Work out the finished part from the listing and answer in its coordinate system (mm). Face numbers are marked on the shaded views. Round coordinates to 2 decimals unless told otherwise and drop trailing zeros. Order: outer loops, then holes, each group sorted by start corner. A loop starts at its lowest first (then second) coordinate and runs counter-clockwise, first axis right, second up. Notation, with made-up numbers: (13, -25) -> (20, -25) arc R6 ccw to (20, -18) -> close; hole circle Ø4 at (81, -8.5). An arc over 180 degrees is marked (long way). Use one line per item in the form item = value.
```python
from build123d import *

# Parameters (mm, degrees)
REVOLVE2_ANGLE           = 7.5
SKETCH4_W                = 33.25
SKETCH4_H                = 13
CUT_EXTRUDE5_DEPTH       = 19
SKETCH7_W                = 33.25
SKETCH7_H                = 13
CUT_EXTRUDE7_DEPTH       = 19
CUT_EXTRUDE8_DEPTH       = 1799.499288206
CUT_EXTRUDE8_DEPTH_BACK  = 1799.499288206
SKETCH9_W                = 188.635889627
SKETCH9_H                = 632.041441351
CUT_EXTRUDE9_DEPTH       = 1799.499288206
CUT_EXTRUDE9_DEPTH_BACK  = 1799.499288206
SKETCH10_W               = 436.927860133
SKETCH10_H               = 1601.4752783
CUT_EXTRUDE10_DEPTH      = 143.403889156
CUT_EXTRUDE10_DEPTH_BACK = 143.403889156


with BuildPart() as part:
    # Sketch2 → Revolve2 (revolve)
    with BuildSketch(Plane.XY):
        with BuildLine():
            Line((0, 993.075249624), (0, 990.6))
            ThreePointArc((0, 990.6), (990.6, 0), (0, -990.6))
            Line((0, -990.6), (0, -993.075249624))
            ThreePointArc((0, -993.075249624), (357.30221933, -926.570869107), (666.748724276, -735.965073963))
            Line((666.748724276, -735.965073963), (742.973100692, -735.965073963))
            Line((742.973100692, -735.965073963), (742.973100692, -658.930514596))
            ThreePointArc((742.973100692, -658.930514596), (993.075236283, 0.162783709), (742.757038562, 659.174053709))
            Line((742.757038562, 659.174053709), (742.757038562, 722.715073963))
            Line((742.757038562, 722.715073963), (681.088374063, 722.715073963))
            ThreePointArc((681.088374063, 722.715073963), (366.393230651, 923.013787519), (0, 993.075249624))
        make_face()
    revolve(axis=Axis((0, 993.075249624, 0), (0, -1, 0)), revolution_arc=REVOLVE2_ANGLE)

    # Sketch4 → Cut-Extrude5 (cut)
    with BuildSketch(Plane.XZ.offset(735.965073963)):
        with Locations((705.258501449, 49.061390401)):
            Rectangle(SKETCH4_W, SKETCH4_H)
    extrude(amount=-CUT_EXTRUDE5_DEPTH, mode=Mode.SUBTRACT)

    # Sketch7 → Cut-Extrude7 (cut)
    with BuildSketch(Plane(origin=(0, 722.715073963, 0), x_dir=(-1, 0, 0), z_dir=(0, 1, 0))):
        with Locations((-714.999743141, 46.422731407)):
            Rectangle(SKETCH7_W, SKETCH7_H)
    extrude(amount=-CUT_EXTRUDE7_DEPTH, mode=Mode.SUBTRACT)

    # Sketch9 → Cut-Extrude8 (cut, two sides: drawn at the far end of the back side and taken through both)
    with BuildSketch(Plane(origin=(770.075395243, 627.042532096, 0), x_dir=(0, 0, -1), z_dir=(0.775445159402277, 0.6314149228198344, 0)).offset(-CUT_EXTRUDE8_DEPTH_BACK)):
        with Locations((-24.021749008, 516.225121034)):
            Rectangle(SKETCH9_W, SKETCH9_H)
    extrude(amount=CUT_EXTRUDE8_DEPTH + CUT_EXTRUDE8_DEPTH_BACK, mode=Mode.SUBTRACT)

    # Sketch10 → Cut-Extrude9 (cut, two sides: drawn at the far end of the back side and taken through both)
    with BuildSketch(Plane(origin=(770.075395243, 627.042532096, 0), x_dir=(0, 0, -1), z_dir=(0.775445159402277, 0.6314149228198344, 0)).offset(-CUT_EXTRUDE9_DEPTH_BACK)):
        with Locations((4.82975611, -781.418075933)):
            Rectangle(SKETCH10_W, SKETCH10_H)
    extrude(amount=CUT_EXTRUDE9_DEPTH + CUT_EXTRUDE9_DEPTH_BACK, mode=Mode.SUBTRACT)

    # Sketch12 → Cut-Extrude10 (cut, two sides: drawn at the far end of the back side and taken through both)
    with BuildSketch(Plane(origin=(700.633749088, 703.783206005, 0), x_dir=(0.7086907122814721, -0.7055192940848463, 0), z_dir=(0.7055192940848463, 0.7086907122814721, 0)).offset(-CUT_EXTRUDE10_DEPTH_BACK)):
        with BuildLine():
            Line((-41.294583605, -87.970897636), (-47.210429628, -112.285313767))
            Line((-47.210429628, -112.285313767), (-119.119874742, -100.128105701))
            Line((-119.119874742, -100.128105701), (-110.576768671, 17.662490687))
            Line((-110.576768671, 17.662490687), (-37.208423865, 15.148795667))
            Line((-37.208423865, 15.148795667), (-37.208423865, 0))
            add(Edge.make_bspline(
                [(-41.294583605, -87.970897636), (-39.934567915, -73.394235927), (-38.912646446, -58.753764388), (-37.549574236, -29.408857228), (-37.208423865, -14.704430952), (-37.208423865, 0)],
                knots=[0, 0, 0, 0, 0.5, 0.5, 1, 1, 1, 1], degree=3))
        make_face()
        with BuildLine():
            add(Edge.make_bspline(
                [(66.778461717, -97.878222384), (68.291902553, -81.657148428), (69.428925425, -65.367159938), (70.945475233, -32.718109498), (71.325001659, -16.35905716), (71.325001659, 0)],
                knots=[0, 0, 0, 0, 0.5, 0.5, 1, 1, 1, 1], degree=3))
            Line((71.325001659, 0), (71.325001659, 10.254449573))
            Line((71.325001659, 10.254449573), (98.450701035, 7.723597346))
            Line((98.450701035, 7.723597346), (86.999767635, -115.007620888))
            Line((86.999767635, -115.007620888), (65.180273381, -115.007620888))
            Line((65.180273381, -115.007620888), (66.778461717, -97.878222384))
        make_face()
    extrude(amount=CUT_EXTRUDE10_DEPTH + CUT_EXTRUDE10_DEPTH_BACK, mode=Mode.SUBTRACT)


solid = part.part
```
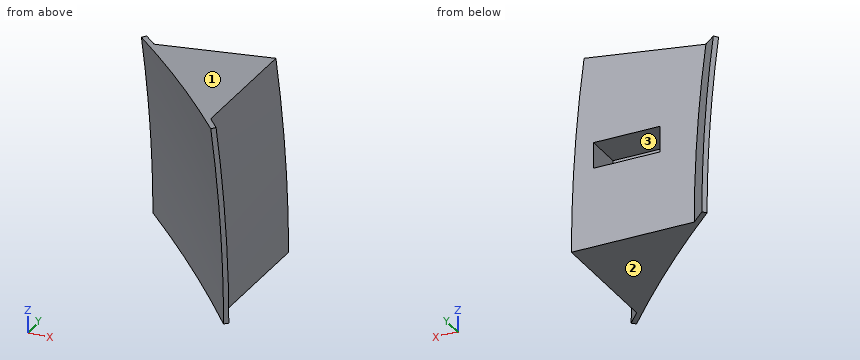
Item 1: Flat-ended cylindrical pins translate along their axes: P1, Ø14.5, axis at y = 717, z = 47.5, coming from the -X side; P2, Ø14.5, axis at y = 709, z = 47, coming from the +X side; P3, Ø5.5, axis at x = 712.5, y = 714.5, coming from the +Z side. Find the tip coordinate at first contact, or state that the pin passes through.
Findings:
P1 = 674.14
P2 = 741.69
P3 = 94.16
Item 2: Consider line 1 along Z through (x, y) = (700.5, 717); line 2 along X through (y, z) = (686.5, 44); line 3 along X through (y, z) = (704.5, 5). Determine where each line is inside the solid, lowest interval first.
Findings:
line_1 = 0 to 39.92, 52.92 to 92.22
line_2 = 712.79 to 741.45
line_3 = 696.38 to 742.74
Item 3: The part is cut by section D-D, the plane x = 705. Give the vertices of the cut face in (y, z).
Findings:
outline = (689.67, 92.82) arc R695.89 cw to (695.89, 0) -> (722.72, 0) -> (722.72, 39.92) -> (703.72, 39.92) -> (703.72, 52.92) -> (722.72, 52.92) -> (722.72, 92.82) -> close
Item 4: The part is cut by section A-A, the plane y = 708.5. Give the vertices of the cut face in (x, z), and give its area (3 significant figures).
Findings:
outline = (686.4, 90.37) arc R692.33 cw to (692.33, 0) -> (742.76, 0) arc R742.76 ccw to (736.4, 96.95) -> close; hole (698.37, 39.92) -> (731.62, 39.92) -> (731.62, 52.92) -> (698.37, 52.92) -> close
area = 4,300 mm^2
Item 5: Determine the mould class of the marked faces 1, 2 and 3 for opening direction X: released by +X, released by -X, zero draft, split by the parting line, or undercut.
Findings:
face_1 = released by -X
face_2 = zero draft
face_3 = undercut
Item 6: The part is cut by section C-C, the plane y = 721. Give the vertices of the cut face in (x, z), and give its area (3 significant figures).
Findings:
outline = (673.49, 88.67) arc R679.3 cw to (679.3, 0) -> (742.76, 0) arc R742.76 ccw to (736.4, 96.95) -> close; hole (698.37, 39.92) -> (731.62, 39.92) -> (731.62, 52.92) -> (698.37, 52.92) -> close
area = 5,470 mm^2
Item 7: The part is cut by section B-B, the plane x = 724. Give the vertices of the cut face in (y, z), and give its area (3 significant figures).
Findings:
outline = (669.35, 95.32) arc R676.1 cw to (676.1, 0) -> (722.72, 0) -> (722.72, 39.92) -> (703.72, 39.92) -> (703.72, 52.92) -> (722.72, 52.92) -> (722.72, 95.32) -> close
area = 4,410 mm^2
